from build123d import *

# Parameters (mm, degrees)
SKETCH1_R          = 3.96875
EXTRUDE1_DEPTH     = 3.96875
SKETCH2_W          = 1.905
SKETCH2_H          = 7.9375
CUT_EXTRUDE1_DEPTH = 1.5875
SKETCH4_R          = 2.38125
EXTRUDE2_DEPTH     = 3.175
SKETCH5_R          = 2.0828
EXTRUDE3_DEPTH     = 4.7625
CHAMFER1_SIZE      = 0.508
CHAMFER2_SIZE      = 0.47625


with BuildPart() as part:
    # Sketch1 → Extrude1 (new body)
    with BuildSketch(Plane(origin=(0, 0, 0), x_dir=(1, 0, 0), z_dir=(0, 1, 0))):
        Circle(SKETCH1_R)
    extrude(amount=EXTRUDE1_DEPTH)

    # Sketch2 → Cut-Extrude1 (cut)
    with BuildSketch(Plane(origin=(0, 3.96875, 0), x_dir=(-1, 0, 0), z_dir=(0, 1, 0))):
        Rectangle(SKETCH2_W, SKETCH2_H)
    extrude(amount=-CUT_EXTRUDE1_DEPTH, mode=Mode.SUBTRACT)

    # Sketch4 → Extrude2 (add)
    with BuildSketch(Plane.XZ):
        Circle(SKETCH4_R)
    extrude(amount=EXTRUDE2_DEPTH)

    # Sketch5 → Extrude3 (add)
    with BuildSketch(Plane.XZ.offset(3.175)):
        Circle(SKETCH5_R)
    extrude(amount=EXTRUDE3_DEPTH)

    # Chamfer1
    chamfer1_edges = [part.edges().sort_by_distance(p)[0] for p in [
        (3.124996875, 3.96875, -2.446501807),
        (-3.96875, 3.96875, 0),
    ]]
    chamfer(chamfer1_edges, length=CHAMFER1_SIZE)

    # Chamfer2
    chamfer2_edges = [part.edges().sort_by_distance(p)[0] for p in [
        (-2.0828, -7.9375, 0),
    ]]
    chamfer(chamfer2_edges, length=CHAMFER2_SIZE)


solid = part.part
The model under review builds one solid part; all positions refer to its coordinate system, in mm. A direction names the side the tool comes from. Round coordinates to 2 decimals unless told otherwise and drop trailing zeros. Loops run counter-clockwise (first coordinate to the right, second up) from the corner with the lowest first, then second, coordinate; pieces in that order, holes last. Notation, with made-up numbers: (70, 49.5) - (90, 49.5) arc R20 cw to (90, 83.5) - close; hole circle Ø11 at (3, 62.25). An arc over 180 degrees is marked (long way). Use CSV: the item, a comma, the result in double quotes.
(1) For line 1 (Y direction, x = -3, z = 0); line 2 (Y direction, x = 2, z = -1) (3 decimals); line 3 (Z direction, x = 1.5, y = -5.25), list the stretches that pass through material, from the lowest coordinate up.
Working result:
line 1,"y = 0 to 3.97"
line 2,"y = -3.175 to 3.969"
line 3,"z = -1.45 to 1.45"
(2) Take a section at D-D, the plane y = -2.25. Give the boundary of the cut face in (x, z).
Working result:
outline,"circle Ø4.76 at (0, 0)"
(3) Clearance check with flat-ended pins moving along their axes: P1, Ø1.5, axis at y = 1.5, z = -2.5, coming from the -X side; P2, Ø1.7, axis at y = 3.5, z = -1.5, coming from the +X side (3 decimals); P3, Ø1.7, axis at y = 3.5, z = -1, coming from the -X side; P4, Ø2, axis at x = 0, z = -2, coming from the +Y side. State where each tip first meets the part, or that it passes through.
Working result:
P1,"stops at x = -3.56"
P2,"stops at x = 3.915"
P3,"stops at x = -3.97"
P4,"stops at y = 3.97"
(4) Machinability: for faces 1 (the flat face through (2, 3.969, 0)), 2 (the flat face through (0, 2.381, 0)), 3 (the cylindrical face through (1.987, -5.288, 0.626)), which of the approach directions +Z, -Z, +X, -X, +Y, -Y give a long, thin tool a straight path to every point of the face, cutting with its end or side? Answer none if there is none.
Working result:
face 1,"+Z, -Z, +X, -X, +Y"
face 2,"+Z, -Z, +Y"
face 3,"-Y"
(5) Take a section at C-C, the plane y = -4.5. Give the boundary of the cut face in (x, z), plus the area to 3 significant figures.
Working result:
outline,"circle Ø4.17 at (0, 0)"
area,"13.6 mm^2"
